Can you work these out from the model? Positions are in its coordinate system, mm. Give positions to 0.01 mm unless a question says otherwise; leave off trailing zeros. Order: outer loops, then holes, each group sorted by start corner. A loop starts at its lowest first (then second) coordinate and runs counter-clockwise, first axis right, second up. Notation, with made-up numbers: M 3,19 L 8,19 A24 cw 8,44 Z; hole C 66,-33.75 d8. An arc over 180 degrees is marked long. Use one line per item in the form item = value. Start each with the question number.
1. I want a section at C-C, the plane x = 57.5. List the corners of the cut face in (y, z) for me, and give its area (3 significant figures).
2. I want a section at B-B, the plane z = 0. List the corners of the cut face in (x, y) for me.
3. I want a section at D-D, the plane x = 5. List the corners of the cut face in (y, z) for me.
4. I want a section at A-A, the plane y = 0. List the corners of the cut face in (x, z) for me.
5. Will these pins go through, and if not, where does the flat tip stop? P1, Ø10, axis at x = 18, z = 7, coming from the +Y side; P2, Ø3, axis at x = 37.5, z = -2.5, coming from the +Y side; P3, Ø1.5, axis at x = -33.5, y = 0, coming from the +Z side; P4, Ø1, axis at x = 9.5, z = -4, coming from the +Y side.
6. I need wall thicknesses on L1, parallel to X at y = 0, z = -8.45; L2, parallel to Z at x = 20.5, y = 0; L3, parallel to Z at x = 22.5, y = 5.25. Which ranges of each line are inside material? Lowest first, please.
Autodesk Inventor part; units mm, degrees
ref_plane "MidSidePlane" through (0, 0, 10) normal (0, 0, 1) x (1, 0, 0)
ref_plane "YZ Plane" through (0, 0, 0) normal (1, 0, 0) x (0, 1, 0)
ref_plane "XZ Plane" through (0, 0, 0) normal (0, 1, 0) x (-1, 0, 0)
sketch "ShaftProfile" plane through (0, 0, 0) normal (0, 0, 1) x (1, 0, 0)
  line L0 (-58, 0) -> (82, 0) construction
  line L1 (-38, 9) -> (62, 9)
  line L2 (62, 9) -> (62, 0)
  line L3 (-38, 0) -> (-38, 9)
  line L4 (-38, 0) -> (62, 0)
  point P0 (0, 0)
  dimension "d1" = 100
  dimension "d2" = 9
  dimension "d4" = 38
revolve "ShaftFeature" add sketch "ShaftProfile" angle 360 about axis through (-38, 0, 0) along (1, 0, 0)
sketch "Sketch2" plane through (-38, 0, 0) normal (-1, 0, 0) x (0, 0, 1)
  circle A0 centre (0, 0) radius 9
hole "ShaftHoleFeature" at (-38, 0, 0) direction (1, 0, 0) diameter 16 end through all
ref_plane "MidSidePlane" through (0, 0, 10) normal (0, 0, 1) x (1, 0, 0)
sketch "CapHoles" plane through (0, 0, 10) normal (0, 0, 1) x (1, 0, 0)
  line L0 (62, -9) -> (62, 9) construction
  line L1 (-38, -9) -> (-38, 9) construction
  line L2 (-48, 0) -> (22, 0) construction
  circle A0 centre (-33.5, 0) radius 1.25
  circle A1 centre (57.5, 0) radius 1.25
  dimension "d24" = 2.5
  dimension "d25" = 4.5
  dimension "d26" = 4.5
extrude "CapHolesFeature" cut sketch "CapHoles" against normal through all
equation "\"d26\" = d25"
properties part number "BackPair1PistonShaft"
Check result:
q1.outline = M -1.25,-8.91 L -1.25,-7.9 A8 cw -1.25,7.9 L -1.25,8.91 A9 ccw Z; M 1.25,-8.91 A9 ccw 1.25,8.91 L 1.25,7.9 A8 cw 1.25,-7.9 Z
q1.area = 48.4 mm2
q2.outline = M -38,-9 L 62,-9 L 62,-8 L -38,-8 Z; M -38,8 L 62,8 L 62,9 L -38,9 Z
q3.outline = C 0,0 d18; hole C 0,0 d16
q4.outline = M -38,-9 L -34.75,-9 L -34.75,-8 L -38,-8 Z; M -38,8 L -34.75,8 L -34.75,9 L -38,9 Z; M -32.25,-9 L 56.25,-9 L 56.25,-8 L -32.25,-8 Z; M -32.25,8 L 56.25,8 L 56.25,9 L -32.25,9 Z; M 58.75,-9 L 62,-9 L 62,-8 L 58.75,-8 Z; M 58.75,8 L 62,8 L 62,9 L 58.75,9 Z
q5.P1 = 8.77
q5.P2 = 8.94
q5.P3 = through
q5.P4 = 8.29
q6.L1 = -38 to -34.75, -32.25 to 56.25, 58.75 to 62
q6.L2 = -9 to -8, 8 to 9
q6.L3 = -7.31 to -6.04, 6.04 to 7.31
